For this review, use the dimensioned drawing (mm, ordinates from the lowest corner) and the shaded views. A direction names the side the tool comes from. Coordinates: 2 decimals unless noted, no trailing zeros. Write each loop counter-clockwise with the first axis right and the second up, starting at its lowest first coordinate (ties: lowest second). Pieces come first, ordered by that corner, then holes.
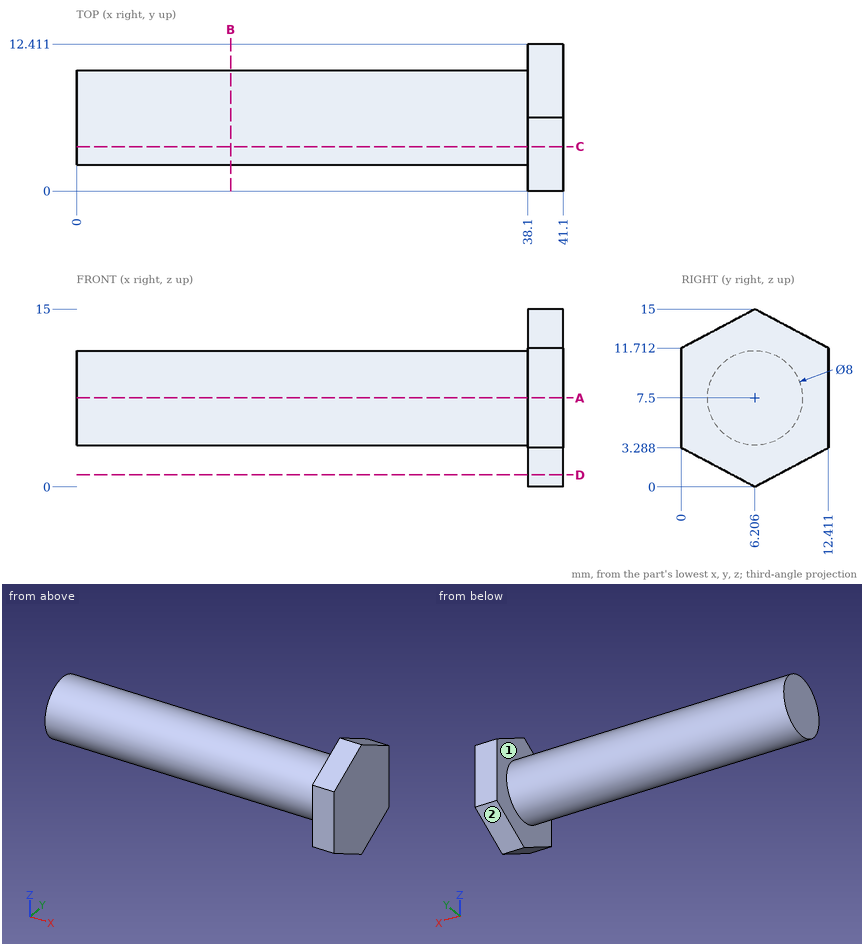
Item 1: Take a section at D-D, the plane z = 1. Write out the cut boundary in (x, y), plus the area to 3 significant figures.
Solved:
outline: (38.1, 4.32) - (41.1, 4.32) - (41.1, 8.09) - (38.1, 8.09) - close
area: 11.3 mm2
Item 2: Take a section at B-B, the plane x = 13. Write out the cut boundary in (y, z) (1 decimal).
Solved:
outline: circle Ø8 at (6.2, 7.5)
Item 3: Take a section at C-C, the plane y = 3.75. Write out the cut boundary in (x, z), plus the area to 3 significant figures.
Solved:
outline: (0, 4.34) - (38.1, 4.34) - (38.1, 1.3) - (41.1, 1.3) - (41.1, 13.7) - (38.1, 13.7) - (38.1, 10.66) - (0, 10.66) - close
area: 278 mm2
Item 4: Machinability: for the marked faces 1 and 2, which of the approach directions +Z, -Z, +X, -X, +Y, -Y give a long, thin tool a straight path to every point of the face, cutting with its end or side? Answer none if there is none.
Solved:
face 1: -X
face 2: -Z, +X, -X, +Y
Item 5: Take a section at A-A, the plane z = 7.5. Write out the cut boundary in (x, y) (1 decimal), plus the area to 3 significant figures.
Solved:
outline: (0, 2.2) - (38.1, 2.2) - (38.1, 0) - (41.1, 0) - (41.1, 12.4) - (38.1, 12.4) - (38.1, 10.2) - (0, 10.2) - close
area: 342 mm2
Item 6: To check wall thickness, follow line 1 along X through (y, z) = (1.25, 11.75); line 2 along Z through (x, y) = (16, 6.25); line 3 along Z through (x, y) = (17, 7.75). State the ranges of each line that lie inside material, in increasing order.
Solved:
line 1: x = 38.1 to 41.1
line 2: z = 3.5 to 11.5
line 3: z = 3.81 to 11.19
Item 7: For pin 1 (5 mm diameter, centred on x = 30, y = 8.5, fed in from -Z); pin 2 (3 mm diameter, centred on x = 34.5, z = 10, fed in from -Y); pin 3 (8 mm diameter, centred on x = 9, z = 2, fed in from +Y); pin 4 (3 mm diameter, centred on y = 4.5, z = 2.5, fed in from -X), all flat-tipped, find the tip position at first contact; note any pin that passes through.
Solved:
pin 1: stops at z = 3.5
pin 2: stops at y = 2.33
pin 3: stops at y = 9.91
pin 4: stops at x = 0
